from build123d import *
from build123d.topology import SkipClean

# Parameters (mm, degrees)
SKETCH1_R           = 25.25
BOSS_EXTRUDE1_DEPTH = 12.7
SKETCH2_R           = 18.9
BOSS_EXTRUDE2_DEPTH = 25.4
SKETCH3_R           = 4.5
CUT_EXTRUDE1_DEPTH  = 13
CUT_EXTRUDE2_DEPTH  = 20
SKETCH5_R           = 2.575
CUT_EXTRUDE3_DEPTH  = 5


with BuildPart() as part:
    # Sketch1 → Boss-Extrude1 (new body)
    with BuildSketch(Plane.XY):
        Circle(SKETCH1_R)
    extrude(amount=-BOSS_EXTRUDE1_DEPTH)

    # Sketch2 → Boss-Extrude2 (add)
    with BuildSketch(Plane(origin=(0, 0, -12.7), x_dir=(-1, 0, 0), z_dir=(0, 0, -1))):
        with Locations(Location((0, 0, 0), (0, 0, 180))):
            Circle(SKETCH2_R)
    extrude(amount=BOSS_EXTRUDE2_DEPTH)

    # Sketch3 → Cut-Extrude1 (cut)
    with BuildSketch(Plane(origin=(0, 0, -38.1), x_dir=(-1, 0, 0), z_dir=(0, 0, -1))):
        Circle(SKETCH3_R)
    extrude(amount=-CUT_EXTRUDE1_DEPTH, mode=Mode.SUBTRACT)

    # Sketch4 → Cut-Extrude2 (cut)
    with BuildSketch(Plane.XY):
        with BuildLine():
            Line((-2.24, 1.270049212), (2.24, 1.270049212))
            ThreePointArc((2.24, 1.270049212), (0, -2.575), (-2.24, 1.270049212))
        make_face()
    extrude(amount=-CUT_EXTRUDE2_DEPTH, mode=Mode.SUBTRACT)

    # Sketch5 → Cut-Extrude3 (cut)
    with SkipClean():  # the faces are left unmerged after this step: merging them gives an invalid solid
        with BuildSketch(Plane.XY):
            Circle(SKETCH5_R)
        extrude(amount=-CUT_EXTRUDE3_DEPTH, mode=Mode.SUBTRACT)


solid = part.part
The model under review builds one solid part; all positions refer to its coordinate system, in mm. A direction names the side the tool comes from. Coordinates: 2 decimals unless noted, no trailing zeros. Write each loop counter-clockwise with the first axis right and the second up, starting at its lowest first coordinate (ties: lowest second). Pieces come first, ordered by that corner, then holes. Notation, with made-up numbers: (89.5, 68.5) - (95.5, 68.5) arc R15 ccw to (95.5, 92.5) - close; hole circle Ø11 at (29.25, 75). An arc over 180 degrees is marked (long way). Answer as a JSON object with one key per item and string values. Group by question number.
1. Machinability: for faces 4 (the face through (0, -5, 0)), 5 (the face through (0, 2, -5)), 6 (the face through (0, 0, -25.1)), which of the approach directions +Z, -Z, +X, -X, +Y, -Y give a long, thin tool a straight path to every point of the face, cutting with its end or side? Answer none if there is none.
2. Add section C-C (z = -33). Give the boundary of the cut face in (x, y).
3. Add section A-A (x = 0). Give the boundary of the cut face in (y, z) (3 decimals).
4. Mouldability with a two-part tool opening along Y and no side actions: class faces 1 (the face through (0.59, 4.46, -31.69)), 2 (the face through (18.027, -5.677, -25.222)), 3 (the face through (4, -19, -12.7)) as pulls with the +Y half, pulls with the -Y half, needs draft (parallel to the pull), parting line crosses it, or undercut.
5. To check wall thickness, follow probe 1 along Y at (x, z) = (0, -33.25); probe 2 along Z at (x, y) = (-21, -4); probe 3 along Z at (x, y) = (-4, 1). State the ranges of each line that lie inside material, in increasing order.
6. Add section B-B (y = 0). Give the boundary of the cut face in (x, z) (3 decimals), plus the area to 3 significant figures.
7. Add section D-D (y = -16). Give the boundary of the cut face in (x, z), plus the area to 3 significant figures.
8. Clearance check with flat-ended pins moving along their axes: pin 1 Ø6 at (x, z) = (1, -33.5) entering from -Y; pin 2 Ø8 at (x, y) = (16.5, -17.5) entering from -Z; pin 3 Ø2 at (y, z) = (11, -33) entering from -X. State where each tip first meets the part, or that it passes through.
Findings:
{
 "1": {"face 4": "+Z, +X, -X, +Y, -Y", "face 5": "+Z", "face 6": "-Z"},
 "2": {"outline": "circle Ø37.8 at (0, 0); hole circle Ø9 at (0, 0)"},
 "3": {"outline": "(-25.25, -12.7) - (-18.9, -12.7) - (-18.9, -38.1) - (-4.5, -38.1) - (-4.5, -25.1) - (4.5, -25.1) - (4.5, -38.1) - (18.9, -38.1) - (18.9, -12.7) - (25.25, -12.7) - (25.25, 0) - (2.575, 0) - (2.575, -5) - (1.27, -5) - (1.27, -20) - (-2.575, -20) - (-2.575, 0) - (-25.25, 0) - close"},
 "4": {"face 1": "undercut", "face 2": "parting line crosses it", "face 3": "needs draft"},
 "5": {"probe 1": "-18.9 to -4.5, 4.5 to 18.9", "probe 2": "-12.7 to 0", "probe 3": "-25.1 to 0"},
 "6": {"outline": "(-25.25, -12.7) - (-18.9, -12.7) - (-18.9, -38.1) - (-4.5, -38.1) - (-4.5, -25.1) - (4.5, -25.1) - (4.5, -38.1) - (18.9, -38.1) - (18.9, -12.7) - (25.25, -12.7) - (25.25, 0) - (2.575, 0) - (2.575, -20) - (-2.575, -20) - (-2.575, 0) - (-25.25, 0) - close", "area": "1,380 mm²"},
 "7": {"outline": "(-19.53, -12.7) - (-10.06, -12.7) - (-10.06, -38.1) - (10.06, -38.1) - (10.06, -12.7) - (19.53, -12.7) - (19.53, 0) - (-19.53, 0) - close", "area": "1,010 mm²"},
 "8": {"pin 1": "y = -18.9", "pin 2": "z = -12.7", "pin 3": "x = -16.04"}
}
